Work out the finished part from the listing and answer in its coordinate system (mm). A direction names the side the tool comes from. Round coordinates to 2 decimals unless told otherwise and drop trailing zeros. Write each loop counter-clockwise with the first axis right and the second up, starting at its lowest first coordinate (ties: lowest second). Pieces come first, ordered by that corner, then holes.
1. Find section B-B (x = 13.25). Write down the section's boundary in (y, z).
2. A tool of negligible diameter and unlimited length cuts with its end or side. For faces 1 (the face through (16, 3, 49)), 2 (the face through (2, 25, 49)), from which of +Z, -Z, +X, -X, +Y, -Y can it reach the whole face along a straight path? Write none if from no direction.
3. Straight lines are drawn through the part: probe 1 along X at (y, z) = (17.5, 13.5); probe 2 along X at (y, z) = (5, 84). For each, find the intervals that lie inside material, in ascending order.
4. Flat-ended cylindrical pins translate along their axes: pin 1 Ø3 at (y, z) = (22, 24) entering from -X; pin 2 Ø5.5 at (x, z) = (18, 27) entering from +Y; pin 3 Ø6 at (x, y) = (21.5, 7) entering from +Z; pin 4 Ø5.5 at (y, z) = (19, 50.5) entering from +X. Find the tip coordinate at first contact, or state that the pin passes through.
5. Find section A-A (z = 24). Write down the section's boundary in (x, y).
Autodesk Fusion 360 part; units mm, degrees
sketch "スケッチ1" plane through (0, 0, 0) normal (0, 0, 1) x (1, 0, 0)
  line L0 (0, 25) -> (0, 0)
  line L1 (3, 7) -> (3, 25)
  arc A0 (3, 7) -> (7, 3) centre (7, 7) ccw
  line L2 (0, 0) -> (25, 0)
  line L3 (25, 3) -> (7, 3)
  line L4 (25, 0) -> (25, 3)
  line L5 (3, 25) -> (0, 25)
extrude "押し出し1" add sketch "スケッチ1" along normal blind 100
Worked answers:
1. outline: (0, 0) - (3, 0) - (3, 100) - (0, 100) - close
2. face 1: +Z, -Z, +X, +Y
2. face 2: +Z, -Z, +X, -X, +Y
3. probe 1: x = 0 to 3
3. probe 2: x = 0 to 3.54
4. pin 1: stops at x = 0
4. pin 2: stops at y = 3
4. pin 3: passes through
4. pin 4: stops at x = 3
5. outline: (0, 0) - (25, 0) - (25, 3) - (7, 3) arc R4 cw to (3, 7) - (3, 25) - (0, 25) - close
